Build history of the part. All positions in model axes, mm. Face numbers are marked on the shaded views. A direction names the side the tool comes from. Give positions to 0.01 mm unless a question says otherwise; leave off trailing zeros. Loops run counter-clockwise (first coordinate to the right, second up) from the corner with the lowest first, then second, coordinate; pieces in that order, holes last. Notation, with made-up numbers: M 4.5,-9.75 L 61.5,-9.75 A13 ccw 61.5,-1.75 Z; hole C 22,52.25 d1. An arc over 180 degrees is marked long. Answer as a JSON object with one key per item and string values. Group by question number.
1. Drill centre lines: line 1 along Y through (x, z) = (2.25, -3.25); line 2 along Y through (x, z) = (0.95, -5.25); line 3 along X through (y, z) = (5.45, -3.65) (3 decimals). Where is each one in solid material? Low to high. Write a range as [from, to].
2. Drop flat-ended pins along their axis: pin 1 Ø0.6 at (x, y) = (1.5, 7) entering from -Z; pin 2 Ø3 at (y, z) = (2.5, -4) entering from -X; pin 3 Ø0.6 at (x, z) = (-0.5, -2) entering from +Y. Give the stop position or say it passes through.
3. Slice it at B-B (z = -3.65). Give the number of separate pieces and of enclosed holes in the cut face, then the cut area to 3 significant figures.
4. Mould opens along X. For the marked faces 3, 4, 5 and 6 say: released by +X, released by -X, zero draft, split by the parting line, or undercut.
5. 3-axis set-ups, long thin cutter, end or side, ignore diameter. For the marked faces 1 and 2: which of +Z, -Z, +X, -X, +Y, -Y reach the whole face in a straight line?
6. Slice it at C-C (z = -0.5). List the corners of the cut face in (x, y).
7. Slice it at A-A (y = 1). List the corners of the cut face in (x, z), then the cut area to 3 significant figures.
8. Slice it at D-D (z = -7). List the corners of the cut face in (x, y), then the cut area to 3 significant figures.
from build123d import *

# Parameters (mm, degrees)
BOSS_EXTRUDE1_DEPTH      = 3.81
CUT_EXTRUDE_1_DEPTH      = 3.01
SKETCH_4_R               = 1.6
CUT_EXTRUDE_2_DEPTH      = 4
SKETCH_7_W               = 1
SKETCH_7_H               = 5.139654773
EXTRUDE_1_DEPTH          = 0.5
SKETCH_8_W               = 1.1
SKETCH_8_H               = 5.189654773
CUT_EXTRUDE_4_DEPTH      = 0.55
SKETCH_10_W              = 0.8
SKETCH_10_H              = 0.5
EXTRUDE_2_DEPTH          = 3
CHAMFER_2_SIZE           = 0.3
CHAMFER_2_SIZE2          = 0.519615242
CHAMFER_3_SIZE           = 0.3
CHAMFER_3_SIZE2          = 0.519615242
CUT_EXTRUDE_START        = 0.2
CUT_EXTRUDE_5_DEPTH      = 0.4
PATTERN_CIRCULAR_1_COUNT = 4


with BuildPart() as part:
    # Sketch1 → Boss-Extrude1 (new body)
    with BuildSketch(Plane(origin=(0, 0, 0), x_dir=(0, 0, -1), z_dir=(1, 0, 0))):
        with BuildLine():
            Line((5.620897226, 8.6), (6.631206986, 4.827492088))
            Line((6.631206986, 4.827492088), (6.7, 4.827492088))
            ThreePointArc((6.7, 4.827492088), (7.124264069, 4.651756157), (7.3, 4.227492088))
            Line((7.3, 4.227492088), (7.3, 0))
            Line((7.3, 0), (0, 0))
            Line((0, 0), (0, 5.59717585))
            Line((0, 5.59717585), (0.656126643, 5.59717585))
            Line((0.656126643, 5.59717585), (1.679102774, 8.6))
            Line((1.679102774, 8.6), (5.620897226, 8.6))
        make_face()
    extrude(amount=BOSS_EXTRUDE1_DEPTH)

    # Sketch 2 → Cut-Extrude 1 (cut)
    with BuildSketch(Plane.ZY.offset(-0.4)):
        Polygon((-7.3, 4.073586509), (-6.032317297, 3.426147995), (-2.931105615, 3.426147995), (-2.931105615, 0.803691629), (-6.262387876, 0.803691629), (-7.3, 0.36356395), align=None)
    extrude(amount=-CUT_EXTRUDE_1_DEPTH, mode=Mode.SUBTRACT)

    # Sketch 4 → Cut-Extrude 2 (cut)
    with BuildSketch(Plane(origin=(0, 8.6, 0), x_dir=(1, 0, 0), z_dir=(0, 1, 0))):
        with Locations(Location((1.905, 3.65, 0), (0, 0, 270))):
            Circle(SKETCH_4_R)
    extrude(amount=-CUT_EXTRUDE_2_DEPTH, mode=Mode.SUBTRACT)

    # Sketch 5 → Revolve 1 (revolve)
    with BuildSketch(Plane.ZY.offset(-1.905), mode=Mode.PRIVATE) as revolve_1_sk:
        with BuildLine():
            Line((-3.65, 7.6), (-4.25, 7.6))
            ThreePointArc((-4.25, 7.6), (-4.957106781, 7.307106781), (-5.25, 6.6))
            Line((-5.25, 6.6), (-5.25, 5.694446069))
            Line((-5.25, 5.694446069), (-3.65, 5.694446069))
            Line((-3.65, 5.694446069), (-3.65, 7.6))
        make_face()
    revolve(revolve_1_sk.sketch.rotate(Axis((1.905, 7.6, -3.65), (0, -1, 0)), 180), axis=Axis((1.905, 7.6, -3.65), (0, -1, 0)))

    # Sketch 7 → Extrude 1 (add)
    with BuildSketch(Plane.ZY):
        with Locations((-1.7, 2.569827387)):
            Rectangle(SKETCH_7_W, SKETCH_7_H)
    extrude(amount=EXTRUDE_1_DEPTH)

    # Sketch 8 → Cut-Extrude 4 (cut)
    with BuildSketch(Plane(origin=(3.81, 0, 0), x_dir=(0, 0, -1), z_dir=(1, 0, 0))):
        with Locations((1.7, 2.594827386)):
            Rectangle(SKETCH_8_W, SKETCH_8_H)
    extrude(amount=-CUT_EXTRUDE_4_DEPTH, mode=Mode.SUBTRACT)

    # Sketch 10 → Extrude 2 (add)
    with BuildSketch(Plane(origin=(0, 0, 0), x_dir=(-1, 0, 0), z_dir=(0, -1, 0))):
        with Locations((-1.905, 3.65)):
            Rectangle(SKETCH_10_W, SKETCH_10_H)
    extrude(amount=EXTRUDE_2_DEPTH)

    # Chamfer 2
    chamfer_2_edges = [part.edges().sort_by_distance(p)[0] for p in [
        (1.505, -3, -3.65),
    ]]
    chamfer_2_side = [part.faces().sort_by_distance(p)[0] for p in [
        (1.905, -3, -3.65),
    ]]
    chamfer(chamfer_2_edges, length=CHAMFER_2_SIZE, length2=CHAMFER_2_SIZE2, reference=chamfer_2_side[0])

    # Chamfer 3
    chamfer_3_edges = [part.edges().sort_by_distance(p)[0] for p in [
        (2.305, -3, -3.65),
    ]]
    chamfer_3_side = [part.faces().sort_by_distance(p)[0] for p in [
        (2.055, -3, -3.65),
    ]]
    chamfer(chamfer_3_edges, length=CHAMFER_3_SIZE, length2=CHAMFER_3_SIZE2, reference=chamfer_3_side[0])

    # Sketch 11 → Cut-Extrude 5 (cut)
    with BuildSketch(Plane.ZY.offset(-1.905).offset(CUT_EXTRUDE_START)):
        Polygon((-4.909756217, 7.996241993), (-3.65, 7.996241993), (-3.65, 6.851621262), (-3.85, 6.851621262), (-4.909756217, 7.607858699), align=None)
    cut_extrude_5 = extrude(amount=-CUT_EXTRUDE_5_DEPTH, mode=Mode.SUBTRACT)

    # Pattern Circular 1: Cut-Extrude 5 ×4 about axis
    pattern_circular_1_axis = Axis((1.905, 0, -3.65), (0, 1, 0))
    for i in range(1, PATTERN_CIRCULAR_1_COUNT):
        add(cut_extrude_5.rotate(pattern_circular_1_axis, i * 360 / PATTERN_CIRCULAR_1_COUNT), mode=Mode.SUBTRACT)


solid = part.part
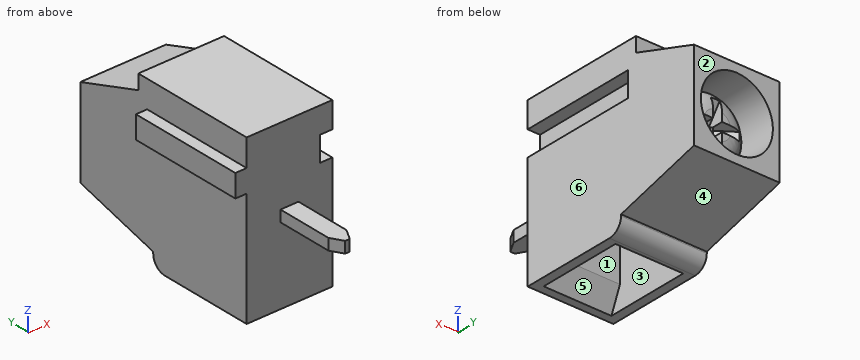
Established:
{
 "1": {"line 1": "y = [0, 0.8], [3.43, 4.6], [5.69, 7.6]", "line 2": "y = [0, 0.8], [3.43, 8.6]", "line 3": "x = [0, 0.305], [3.505, 3.81]"},
 "2": {"pin 1": "stops at z = -6.13", "pin 2": "stops at x = 0", "pin 3": "stops at y = 5.14"},
 "3": {"separate pieces": "1", "enclosed holes": "2", "area": "19.0 mm^2"},
 "4": {"face 3": "undercut", "face 4": "zero draft", "face 5": "undercut", "face 6": "released by +X"},
 "5": {"face 1": "-Z", "face 2": "+Z, -Z, +X, -X, +Y"},
 "6": {"outline": "M 0,0 L 3.81,0 L 3.81,5.6 L 0,5.6 Z"},
 "7": {"outline": "M -0.5,-2.2 L 0,-2.2 L 0,-7.3 L 0.4,-7.3 L 0.4,-2.93 L 3.41,-2.93 L 3.41,-7.3 L 3.81,-7.3 L 3.81,-2.25 L 3.26,-2.25 L 3.26,-1.15 L 3.81,-1.15 L 3.81,0 L 0,0 L 0,-1.2 L -0.5,-1.2 Z", "area": "14.6 mm^2"},
 "8": {"outline": "M 0,0 L 3.81,0 L 3.81,4.75 L 0,4.75 Z; hole M 0.4,0.49 L 3.41,0.49 L 3.41,3.92 L 0.4,3.92 Z", "area": "7.76 mm^2"}
}
